from build123d import *

# Parameters (mm, degrees)
SKETCH1_R           = 4
SKETCH1_R_2         = 2.25
BOSS_EXTRUDE1_DEPTH = 3


with BuildPart() as part:
    # Sketch1 → Boss-Extrude1 (new body)
    with BuildSketch(Plane(origin=(0, 0, 0), x_dir=(-1, 0, 0), z_dir=(0, 0, -1))):
        Polygon((15, 50), (15, 38), (-15, 38), (-15, 50), (-45, 50), (-45, -50), (45, -50), (45, 50), align=None)
        with Locations(Location((-5, -23, 0), (0, 0, 180))):
            Circle(SKETCH1_R, mode=Mode.SUBTRACT)
        with Locations(Location((40, 45, 0), (0, 0, 180))):
            Circle(SKETCH1_R_2, mode=Mode.SUBTRACT)
        with Locations(Location((-40, 45, 0), (0, 0, 180))):
            Circle(SKETCH1_R_2, mode=Mode.SUBTRACT)
        with Locations(Location((-40, -45, 0), (0, 0, 180))):
            Circle(SKETCH1_R_2, mode=Mode.SUBTRACT)
        with Locations(Location((40, -45, 0), (0, 0, 180))):
            Circle(SKETCH1_R_2, mode=Mode.SUBTRACT)
    extrude(amount=-BOSS_EXTRUDE1_DEPTH)


solid = part.part
For this review, take the finished solid that the model builds, in its own axes (mm). A direction names the side the tool comes from. Give positions to 0.01 mm unless a question says otherwise; leave off trailing zeros. Order: outer loops, then holes, each group sorted by start corner. A loop starts at its lowest first (then second) coordinate and runs counter-clockwise, first axis right, second up. Notation, with made-up numbers: M 72.5,16 L 79.5,16 A21 cw 79.5,36 Z; hole C -1,30 d7. An arc over 180 degrees is marked long. Answer in a Markdown table with one row per item. Add a question column.
(1) Mouldability with a two-part tool opening along Y and no side actions: class faces 1 (the face through (39.71, 42.77, 1.48)), 2 (the face through (45, 1, 1)), 3 (the face through (-30, 50, 1)), 4 (the face through (1, -50, 1)) as +Y half, -Y half, draft (parallel to the pull), parting line (faces both ways), or undercut.
(2) Wall thickness on probe 1 along Y at (x, z) = (40, 0.9); probe 2 along X at (y, z) = (-45, 0.9); probe 3 along X at (y, z) = (45, 1.8): over which ranges is each line inside the solid? List them lowest first. Write a range as [from, to].
(3) For pin 1 (1.5 mm diameter, centred on x = -6, z = 2, fed in from +Y), flat-tipped, find the tip position at first contact; note if it passes through.
(4) Consider section A-A on z = 1.4. State the section outline as (x, y) points.
(5) Consider section D-D on y = -23. State the section outline as (x, z) points, and give its area (3 significant figures).
(6) Consider section C-C on y = 45. State the section outline as (x, z) points.
(7) For faces 5 (the face through (-40.29, 42.77, 1.48)), 6 (the face through (15, 44, 1)), list the 3-axis set-ups (+Z, -Z, +X, -X, +Y, -Y) from which the entire face can be reached by the end or side of a thin tool; tool diameter is ignored.
(8) Consider section B-B on x = 5. State the section outline as (y, z) points, and give its area (3 significant figures).
Evaluation:
| question | item | result |
|---|---|---|
| 1 | face 1 | undercut |
| 1 | face 2 | draft |
| 1 | face 3 | +Y half |
| 1 | face 4 | -Y half |
| 2 | probe 1 | y = [-50, -47.25], [-42.75, 42.75], [47.25, 50] |
| 2 | probe 2 | x = [-45, -42.25], [-37.75, 37.75], [42.25, 45] |
| 2 | probe 3 | x = [-45, -42.25], [-37.75, -15], [15, 37.75], [42.25, 45] |
| 3 | pin 1 | stops at y = 38 |
| 4 | outline | M -45,-50 L 45,-50 L 45,50 L 15,50 L 15,38 L -15,38 L -15,50 L -45,50 Z; hole C -40,-45 d4.5; hole C -40,45 d4.5; hole C 5,-23 d8; hole C 40,-45 d4.5; hole C 40,45 d4.5 |
| 5 | outline | M -45,0 L 1,0 L 1,3 L -45,3 Z; M 9,0 L 45,0 L 45,3 L 9,3 Z |
| 5 | area | 246 mm^2 |
| 6 | outline | M -45,0 L -42.25,0 L -42.25,3 L -45,3 Z; M -37.75,0 L -15,0 L -15,3 L -37.75,3 Z; M 15,0 L 37.75,0 L 37.75,3 L 15,3 Z; M 42.25,0 L 45,0 L 45,3 L 42.25,3 Z |
| 7 | face 5 | +Z, -Z |
| 7 | face 6 | +Z, -Z, +Y |
| 8 | outline | M -50,0 L -27,0 L -27,3 L -50,3 Z; M -19,0 L 38,0 L 38,3 L -19,3 Z |
| 8 | area | 240 mm^2 |
